```python
from build123d import *

# Parameters (mm, degrees)
SKETCH_1_R             = 4
EXTRUDE_1_DEPTH        = 11
SKETCH_2_R             = 17.5
SKETCH_2_R_2           = 4
EXTRUDE_2_DEPTH        = 2
SKETCH_3_R             = 17.5
SKETCH_3_R_2           = 4
EXTRUDE_3_DEPTH        = 2
CHAMFER_1_SIZE         = 0.5
HOLE_WIZARD_M3_1_D     = 2.5
HOLE_WIZARD_M3_1_DEPTH = 5
HOLE_WIZARD_M3_1_TIP   = 0.751075774
HOLE_WIZARD_M3_2_D     = 2.5
HOLE_WIZARD_M3_2_DEPTH = 5
HOLE_WIZARD_M3_2_TIP   = 0.751075774


with BuildPart() as part:
    # 草图1 → 凸台-拉伸1 (new body)
    with BuildSketch(Plane(origin=(0, 0, 0), x_dir=(0, 0, -1), z_dir=(1, 0, 0))):
        with BuildLine():
            Line((-1.285, 14.645), (1.285, 14.645))
            Line((1.285, 14.645), (1.828089361, 15.809658892))
            ThreePointArc((1.828089361, 15.809658892), (2.489654511, 15.719059941), (3.146836974, 15.60078979))
            Line((3.146836974, 15.60078979), (3.303446259, 14.325309519))
            Line((3.303446259, 14.325309519), (5.747661506, 13.531135843))
            Line((5.747661506, 13.531135843), (6.624069572, 14.47096843))
            ThreePointArc((6.624069572, 14.47096843), (7.225258803, 14.180368832), (7.813728981, 13.864806685))
            Line((7.813728981, 13.864806685), (7.568528182, 12.603357932))
            Line((7.568528182, 12.603357932), (9.647701858, 11.092749833))
            Line((9.647701858, 11.092749833), (10.771639701, 11.715758753))
            ThreePointArc((10.771639701, 11.715758753), (11.253604423, 11.253604423), (11.715758753, 10.771639701))
            Line((11.715758753, 10.771639701), (11.092749833, 9.647701858))
            Line((11.092749833, 9.647701858), (12.603357932, 7.568528182))
            Line((12.603357932, 7.568528182), (13.864806685, 7.813728981))
            ThreePointArc((13.864806685, 7.813728981), (14.180368832, 7.225258803), (14.47096843, 6.624069572))
            Line((14.47096843, 6.624069572), (13.531135843, 5.747661506))
            Line((13.531135843, 5.747661506), (14.325309519, 3.303446259))
            Line((14.325309519, 3.303446259), (15.60078979, 3.146836974))
            ThreePointArc((15.60078979, 3.146836974), (15.719059941, 2.489654511), (15.809658892, 1.828089361))
            Line((15.809658892, 1.828089361), (14.645, 1.285))
            Line((14.645, 1.285), (14.645, -1.285))
            Line((14.645, -1.285), (15.809658892, -1.828089361))
            ThreePointArc((15.809658892, -1.828089361), (15.719059941, -2.489654511), (15.60078979, -3.146836974))
            Line((15.60078979, -3.146836974), (14.325309519, -3.303446259))
            Line((14.325309519, -3.303446259), (13.531135843, -5.747661506))
            Line((13.531135843, -5.747661506), (14.47096843, -6.624069572))
            ThreePointArc((14.47096843, -6.624069572), (14.180368832, -7.225258803), (13.864806685, -7.813728981))
            Line((13.864806685, -7.813728981), (12.603357932, -7.568528182))
            Line((12.603357932, -7.568528182), (11.092749833, -9.647701858))
            Line((11.092749833, -9.647701858), (11.715758753, -10.771639701))
            ThreePointArc((11.715758753, -10.771639701), (11.253604423, -11.253604423), (10.771639701, -11.715758753))
            Line((10.771639701, -11.715758753), (9.647701858, -11.092749833))
            Line((9.647701858, -11.092749833), (7.568528182, -12.603357932))
            Line((7.568528182, -12.603357932), (7.813728981, -13.864806685))
            ThreePointArc((7.813728981, -13.864806685), (7.225258803, -14.180368832), (6.624069572, -14.47096843))
            Line((6.624069572, -14.47096843), (5.747661506, -13.531135843))
            Line((5.747661506, -13.531135843), (3.303446259, -14.325309519))
            Line((3.303446259, -14.325309519), (3.146836974, -15.60078979))
            ThreePointArc((3.146836974, -15.60078979), (2.489654511, -15.719059941), (1.828089361, -15.809658892))
            Line((1.828089361, -15.809658892), (1.285, -14.645))
            Line((1.285, -14.645), (-1.285, -14.645))
            Line((-1.285, -14.645), (-1.828089361, -15.809658892))
            ThreePointArc((-1.828089361, -15.809658892), (-2.489654511, -15.719059941), (-3.146836974, -15.60078979))
            Line((-3.146836974, -15.60078979), (-3.303446259, -14.325309519))
            Line((-3.303446259, -14.325309519), (-5.747661506, -13.531135843))
            Line((-5.747661506, -13.531135843), (-6.624069572, -14.47096843))
            ThreePointArc((-6.624069572, -14.47096843), (-7.225258803, -14.180368832), (-7.813728981, -13.864806685))
            Line((-7.813728981, -13.864806685), (-7.568528182, -12.603357932))
            Line((-7.568528182, -12.603357932), (-9.647701858, -11.092749833))
            Line((-9.647701858, -11.092749833), (-10.771639701, -11.715758753))
            ThreePointArc((-10.771639701, -11.715758753), (-11.253604423, -11.253604423), (-11.715758753, -10.771639701))
            Line((-11.715758753, -10.771639701), (-11.092749833, -9.647701858))
            Line((-11.092749833, -9.647701858), (-12.603357932, -7.568528182))
            Line((-12.603357932, -7.568528182), (-13.864806685, -7.813728981))
            ThreePointArc((-13.864806685, -7.813728981), (-14.180368832, -7.225258803), (-14.47096843, -6.624069572))
            Line((-14.47096843, -6.624069572), (-13.531135843, -5.747661506))
            Line((-13.531135843, -5.747661506), (-14.325309519, -3.303446259))
            Line((-14.325309519, -3.303446259), (-15.60078979, -3.146836974))
            ThreePointArc((-15.60078979, -3.146836974), (-15.719059941, -2.489654511), (-15.809658892, -1.828089361))
            Line((-15.809658892, -1.828089361), (-14.645, -1.285))
            Line((-14.645, -1.285), (-14.645, 1.285))
            Line((-14.645, 1.285), (-15.809658892, 1.828089361))
            ThreePointArc((-15.809658892, 1.828089361), (-15.719059941, 2.489654511), (-15.60078979, 3.146836974))
            Line((-15.60078979, 3.146836974), (-14.325309519, 3.303446259))
            Line((-14.325309519, 3.303446259), (-13.531135843, 5.747661506))
            Line((-13.531135843, 5.747661506), (-14.47096843, 6.624069572))
            ThreePointArc((-14.47096843, 6.624069572), (-14.180368832, 7.225258803), (-13.864806685, 7.813728981))
            Line((-13.864806685, 7.813728981), (-12.603357932, 7.568528182))
            Line((-12.603357932, 7.568528182), (-11.092749833, 9.647701858))
            Line((-11.092749833, 9.647701858), (-11.715758753, 10.771639701))
            ThreePointArc((-11.715758753, 10.771639701), (-11.253604423, 11.253604423), (-10.771639701, 11.715758753))
            Line((-10.771639701, 11.715758753), (-9.647701858, 11.092749833))
            Line((-9.647701858, 11.092749833), (-7.568528182, 12.603357932))
            Line((-7.568528182, 12.603357932), (-7.813728981, 13.864806685))
            ThreePointArc((-7.813728981, 13.864806685), (-7.225258803, 14.180368832), (-6.624069572, 14.47096843))
            Line((-6.624069572, 14.47096843), (-5.747661506, 13.531135843))
            Line((-5.747661506, 13.531135843), (-3.303446259, 14.325309519))
            Line((-3.303446259, 14.325309519), (-3.146836974, 15.60078979))
            ThreePointArc((-3.146836974, 15.60078979), (-2.489654511, 15.719059941), (-1.828089361, 15.809658892))
            Line((-1.828089361, 15.809658892), (-1.285, 14.645))
        make_face()
        Circle(SKETCH_1_R, mode=Mode.SUBTRACT)
    extrude(amount=EXTRUDE_1_DEPTH)

    # 草图2 → 凸台-拉伸2 (add)
    with BuildSketch(Plane(origin=(11, 0, 0), x_dir=(0, 0, -1), z_dir=(1, 0, 0))):
        Circle(SKETCH_2_R)
        Circle(SKETCH_2_R_2, mode=Mode.SUBTRACT)
    extrude(amount=EXTRUDE_2_DEPTH)

    # 草图3 → 凸台-拉伸3 (add)
    with BuildSketch(Plane.ZY):
        Circle(SKETCH_3_R)
        Circle(SKETCH_3_R_2, mode=Mode.SUBTRACT)
    extrude(amount=EXTRUDE_3_DEPTH)

    # 倒角1
    chamfer_1_edges = [part.edges().sort_by_distance(p)[0] for p in [
        (13, 0, 4),
        (-2, 0, -4),
    ]]
    chamfer(chamfer_1_edges, length=CHAMFER_1_SIZE)

    # M3 螺纹孔1
    with Locations(Plane(origin=(13, 0, 0), x_dir=(0, 0, -1), z_dir=(1, 0, 0))):
        with Locations((-6, 6), (6, 6), (6, -6), (-6, -6)):
            Hole(HOLE_WIZARD_M3_1_D / 2, depth=HOLE_WIZARD_M3_1_DEPTH)
            with Locations((0, 0, -(HOLE_WIZARD_M3_1_DEPTH + HOLE_WIZARD_M3_1_TIP / 2))):  # 118° drill point
                Cone(0, HOLE_WIZARD_M3_1_D / 2, HOLE_WIZARD_M3_1_TIP, mode=Mode.SUBTRACT)

    # M3 螺纹孔2
    with Locations(Plane.ZY.offset(2)):
        with Locations((-6, 6), (6, 6), (6, -6), (-6, -6)):
            Hole(HOLE_WIZARD_M3_2_D / 2, depth=HOLE_WIZARD_M3_2_DEPTH)
            with Locations((0, 0, -(HOLE_WIZARD_M3_2_DEPTH + HOLE_WIZARD_M3_2_TIP / 2))):  # 118° drill point
                Cone(0, HOLE_WIZARD_M3_2_D / 2, HOLE_WIZARD_M3_2_TIP, mode=Mode.SUBTRACT)


solid = part.part
```
Can you work these out from the model? Positions are in its coordinate system, mm. A direction names the side the tool comes from. Coordinates: 2 decimals unless noted, no trailing zeros. Write each loop counter-clockwise with the first axis right and the second up, starting at its lowest first coordinate (ties: lowest second). Pieces come first, ordered by that corner, then holes. Notation, with made-up numbers: M 8.5,-17 L 28.5,-17 A20 ccw 28.5,21 Z; hole C -21,11 d7. An arc over 180 degrees is marked long. Answer as CSV lines item,"result".
Item 1: We'd pull the mould along X, two halves only. Please class faces 4 (the cylindrical face through (5.42, -2.48, -15.72)), 5 (the cylindrical face through (0.54, 4.78, 6.27)), 6 (the conical face through (3.62, 6.15, -6.16)), 7 (the conical face through (7.38, 6.15, 6.16)): +X half, -X half, draft (parallel to the pull), parting line (faces both ways), or undercut.
Geometry results:
face 4,"undercut"
face 5,"draft"
face 6,"-X half"
face 7,"+X half"
Item 2: Imagine slicing it at B-B on x = 11.5. List the corners of the cut face in (y, z) for me, plus the area to 3 significant figures.
Geometry results:
outline,"C 0,0 d35; hole C -6,-6 d2.5; hole C -6,6 d2.5; hole C 0,0 d8; hole C 6,-6 d2.5; hole C 6,6 d2.5"
area,"892 mm2"
Item 3: I'm going to push flat-ended pins straight in: P1, Ø3, axis at x = 7, y = 0, coming from the -Z side; P2, Ø2, axis at x = 9, y = -7, coming from the +Z side; P3, Ø2, axis at y = -6, z = 6, coming from the -X side; P4, Ø6.5, axis at y = 0, z = 0, coming from the -X side. Where does each tip first touch, or does it pass through?
Geometry results:
P1,"stops at z = -15.11"
P2,"stops at z = 14.47"
P3,"stops at x = 3.15"
P4,"passes through"
Item 4: Please list where these lines run through material, in increasing order: line 1 along Z through (x, y) = (10.8, 6); line 2 along X through (y, z) = (-10, 13); line 3 along Y through (x, z) = (-0.55, 0).
Geometry results:
line 1,"z = -13.8 to -7.25, -4.75 to 4.75, 7.25 to 13.8"
line 2,"x = -2 to 0, 11 to 13"
line 3,"y = -17.5 to -4, 4 to 17.5"
Item 5: Imagine slicing it at A-A on z = 0. List the corners of the cut face in (x, y) for me (3 decimals), plus the area to 3 significant figures.
Geometry results:
outline,"M -2,-17.5 L 0,-17.5 L 0,-14.645 L 11,-14.645 L 11,-17.5 L 13,-17.5 L 13,-4.5 L 12.5,-4 L -1.5,-4 L -2,-4.5 Z; M -2,4.5 L -1.5,4 L 12.5,4 L 13,4.5 L 13,17.5 L 11,17.5 L 11,14.645 L 0,14.645 L 0,17.5 L -2,17.5 Z"
area,"342 mm2"
Item 6: On a 3-axis mill with a long thin cutter (end or side, diameter ignored), from which of +Z, -Z, +X, -X, +Y, -Y can I reach the whole of each face in a straight line? I mean faces 1 (the cylindrical face through (10.46, -6.76, 5.01)), 2 (the cylindrical face through (5.42, -11.25, -11.26)), 3 (the cylindrical face through (5.42, 14.18, 7.23)). Say none if no direction works.
Geometry results:
face 1,"+X"
face 2,"-Z, -Y"
face 3,"+Z, +Y"
